from build123d import *

# Parameters (mm, degrees)
SKETCH7_W           = 4.7625
SKETCH7_H           = 2.12122512
BOSS_EXTRUDE2_DEPTH = 53.975
SKETCH8_W           = 2.12122512
SKETCH8_H           = 4.7625
BOSS_EXTRUDE3_DEPTH = 53.975
BOSS_EXTRUDE4_DEPTH = 53.975


with BuildPart() as part:
    # Sketch7 → Boss-Extrude2 (new, symmetric)
    with BuildSketch(Plane.XY):
        with Locations((-4.92125, -2.560612608)):
            Rectangle(SKETCH7_W, SKETCH7_H)
    extrude(amount=BOSS_EXTRUDE2_DEPTH, both=True)



with BuildPart() as body_2:
    # Sketch8 → Boss-Extrude3 (new, symmetric)
    with BuildSketch(Plane.XY):
        with Locations((2.560612608, 4.92125)):
            Rectangle(SKETCH8_W, SKETCH8_H)
    extrude(amount=BOSS_EXTRUDE3_DEPTH, both=True)


with BuildPart() as part_1:
    add(part.part)

    add(body_2.part)  # Boss-Extrude4 merges body 2
    # Sketch11 → Boss-Extrude4 (add, symmetric)
    with BuildSketch(Plane.XY):
        with BuildLine():
            Line((-2.54, -1.500000048), (-7.3025, -1.500000048))
            Line((-7.3025, -1.500000048), (-7.3025, -3.621225168))
            Line((-7.3025, -3.621225168), (-2.54, -3.621225168))
            ThreePointArc((-2.54, -3.621225168), (1.816644097, -1.816644097), (3.621225168, 2.54))
            Line((3.621225168, 2.54), (3.621225168, 7.3025))
            Line((3.621225168, 7.3025), (1.500000048, 7.3025))
            Line((1.500000048, 7.3025), (1.500000048, 2.54))
            Line((1.500000048, 2.54), (-1.500000048, 2.54))
            ThreePointArc((-1.500000048, 2.54), (-1.804608982, 1.804608982), (-2.54, 1.500000048))
            Line((-2.54, 1.500000048), (-2.54, -1.500000048))
        make_face()
    extrude(amount=BOSS_EXTRUDE4_DEPTH, both=True)


solid = part_1.part
Here's how the part is built. I have some questions about the finished solid (model axes, mm). A direction names the side the tool comes from. Coordinates: 2 decimals unless noted, no trailing zeros. Order: outer loops, then holes, each group sorted by start corner. A loop starts at its lowest first (then second) coordinate and runs counter-clockwise, first axis right, second up. Notation, with made-up numbers: M 27.25,-27 L 85.25,-27 A24 cw 85.25,1 Z; hole C -0.5,13 d1. An arc over 180 degrees is marked long. Answer as CSV lines item,"result".
Item 1: Imagine slicing it at A-A on z = 26.5. Write out the boundary of the cut face in (x, y), plus the area to 3 significant figures.
Results found:
outline,"M -7.3,-3.62 L -2.54,-3.62 A6.16 ccw 3.62,2.54 L 3.62,7.3 L 1.5,7.3 L 1.5,2.54 L -1.5,2.54 A1.04 cw -2.54,1.5 L -2.54,-1.5 L -7.3,-1.5 Z"
area,"49.2 mm2"
Item 2: For pin 1 (4 mm diameter, centred on x = -2.5, z = 42.5, fed in from +Y); pin 2 (1.5 mm diameter, centred on y = 0, z = 21, fed in from -X); pin 3 (4 mm diameter, centred on y = 5.5, z = -8.5, fed in from -X), each with a flat end and sliding along its axis, tell me the tip position at first contact or that it passes through.
Results found:
pin 1,"y = 2.54"
pin 2,"x = -2.54"
pin 3,"x = 1.5"
Item 3: Imagine slicing it at C-C on y = 6. Write out the boundary of the cut face in (x, z) (3 decimals).
Results found:
outline,"M 1.5,-53.975 L 3.621,-53.975 L 3.621,53.975 L 1.5,53.975 Z"
Item 4: On a 3-axis mill with a long thin cutter (end or side, diameter ignored), from which of +Z, -Z, +X, -X, +Y, -Y can I reach the whole of each face in a straight line? I mean faces 1 (the face through (-5, -1.5, 1)), 2 (the face through (3.621, 5, 1)). Say none if no direction works.
Results found:
face 1,"+Z, -Z, -X, +Y"
face 2,"+Z, -Z, +X, +Y, -Y"
Item 5: Imagine slicing it at B-B on x = -3.5. Write out the boundary of the cut face in (y, z) (3 decimals), plus the area to 3 significant figures.
Results found:
outline,"M -3.621,-53.975 L -1.5,-53.975 L -1.5,53.975 L -3.621,53.975 Z"
area,"229 mm2"
Item 6: If I drill on line 1 (Y direction, x = -6, z = -10.5); line 2 (X direction, y = 4.5, z = -20); line 3 (Y direction, x = 0, z = 37.5), over which ranges is the centre line in solid material (lowest first)?
Results found:
line 1,"-3.62 to -1.5"
line 2,"1.5 to 3.62"
line 3,"-3.07 to 2.54"
